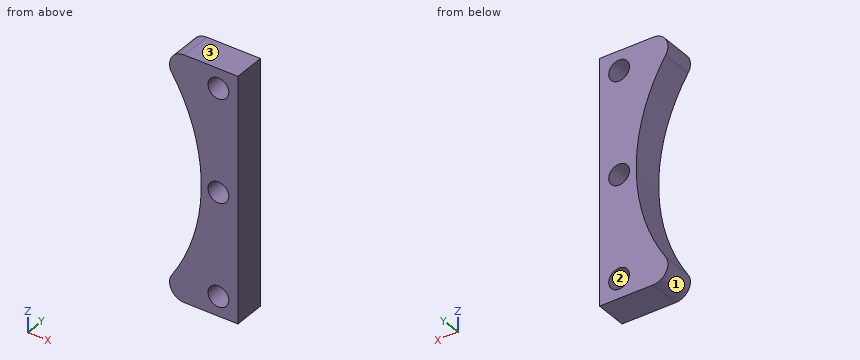
Autodesk Inventor part; units mm, degrees
ref_plane "YZ Plane" through (0, 0, 0) normal (1, 0, 0) x (0, 1, 0)
ref_plane "XZ Plane" through (0, 0, 0) normal (0, 1, 0) x (-1, 0, 0)
ref_plane "XY Plane" through (0, 0, 0) normal (0, 0, 1) x (1, 0, 0)
sketch "Sketch1" plane through (0, 0, 0) normal (0, 1, 0) x (-1, 0, 0)
  arc A0 (-27.9508, 25) -> (-27.9508, -25) centre (0, 0) ccw
  line L0 (-27.9508, 25) -> (-45, 25)
  line L1 (-27.9508, -25) -> (-45, -25)
  line L2 (-45, 25) -> (-45, -25)
  circle A1 centre (-41, 21) radius 2.125
  circle A2 centre (-41, 0) radius 2.125
  circle A3 centre (-41, -21) radius 2.125
  dimension "d0" = 75
  dimension "d3" = 25
  dimension "d4" = 25
  dimension "d5" = 45
  dimension "d6" = 4.25
  dimension "d7" = 4.25
  dimension "d8" = 4.25
  dimension "d9" = 4
  dimension "d10" = 4
  dimension "d11" = 4
  dimension "d12" = 25
  dimension "d13" = 4
  dimension "d14" = 4
extrude "Extrusion1" add sketch "Sketch1" along normal blind 6.5
fillet "Fillet1" radius 3 2 edges at (27.9508, 3.25, 25) (27.9508, 3.25, -25)
properties part number "feeder_stack"
Here's how the part is built. I have some questions about the finished solid (model axes, mm). Face numbers are marked on the shaded views. Round coordinates to 2 decimals unless told otherwise and drop trailing zeros. Order: outer loops, then holes, each group sorted by start corner. A loop starts at its lowest first (then second) coordinate and runs counter-clockwise, first axis right, second up. Notation, with made-up numbers: M 38,89.5 L 90,89.5 A20 ccw 90,103.5 Z; hole C 78.5,84.25 d9. An arc over 180 degrees is marked long. One line per question, with ' | ' between items.
1) I want a section at C-C, the plane y = 1.25. Write out the boundary of the cut face in (x, z) (3 decimals).
Working result:
outline: M 31.485,-20.37 A3 ccw 34.004,-25 L 45,-25 L 45,25 L 34.004,25 A3 ccw 31.485,20.37 A37.5 cw Z; hole C 41,-21 d4.25; hole C 41,0 d4.25; hole C 41,21 d4.25
2) I want a section at A-A, the plane z = 0. Write out the boundary of the cut face in (x, y) (3 decimals), then the cut area to 3 significant figures.
Working result:
outline: M 37.5,0 L 38.875,0 L 38.875,6.5 L 37.5,6.5 Z; M 43.125,0 L 45,0 L 45,6.5 L 43.125,6.5 Z | area: 21.1 mm²
3) I want a section at B-B, the plane x = 41. Write out the boundary of the cut face in (y, z) (3 decimals).
Working result:
outline: M 0,-25 L 6.5,-25 L 6.5,-23.125 L 0,-23.125 Z; M 0,-18.875 L 6.5,-18.875 L 6.5,-2.125 L 0,-2.125 Z; M 0,2.125 L 6.5,2.125 L 6.5,18.875 L 0,18.875 Z; M 0,23.125 L 6.5,23.125 L 6.5,25 L 0,25 Z
4) I need wall thicknesses on line 1 along Z through (x, y) = (41, 6) (3 decimals); line 2 along Z through (x, y) = (40, 2) (3 decimals); line 3 along Z through (x, y) = (32.5, 3). Which ranges of each line are inside material? Lowest first, please.
Working result:
line 1: -25 to -23.125, -18.875 to -2.125, 2.125 to 18.875, 23.125 to 25 | line 2: -25 to -22.875, -19.125 to -1.875, 1.875 to 19.125, 22.875 to 25 | line 3: -24.6 to -18.71, 18.71 to 24.6
5) If we mould it in two halves opening along X, with no side actions, what happens to the marked faces 1, 2 and 3? For each: +X half, -X half, draft (parallel to the pull), parting line (faces both ways), or undercut.
Working result:
face 1: -X half | face 2: undercut | face 3: draft
6) I want a section at D-D, the plane x = 33. Write out the boundary of the cut face in (y, z), then the cut area to 3 significant figures.
Working result:
outline: M 0,-24.83 L 6.5,-24.83 L 6.5,-17.81 L 0,-17.81 Z; M 0,17.81 L 6.5,17.81 L 6.5,24.83 L 0,24.83 Z | area: 91.2 mm²
7) For pin 1 Ø4 at (x, z) = (41, 17.5) entering from -Y, with a flat end and sliding along its axis, tell me the tip position at first contact or that it passes through.
Working result:
pin 1: y = 0
